Read the model definition and answer for the solid it produces. Units are mm, in the model's axes. Coordinates: 2 decimals unless noted, no trailing zeros. Loops run counter-clockwise (first coordinate to the right, second up) from the corner with the lowest first, then second, coordinate; pieces in that order, holes last. Notation, with made-up numbers: M 70,5 L 127,5 A9 cw 127,17 Z; hole C -29,-19.75 d10. An arc over 180 degrees is marked long. Use one line per item in the form item = value. Start each with the question number.
1. A flat-ended cylindrical pin translates along its axis: pin 1 (4 mm diameter, centred on x = 0, y = 0, fed in from +Z) (3 decimals). Find the tip coordinate at first contact, or state that the pin passes through.
2. The part is cut by section B-B (y = 0). Give the vertices of the cut face in (x, z) (1 decimal), plus the area to 3 significant figures.
3. The part is cut by section A-A (x = 0). Give the vertices of the cut face in (y, z) (1 decimal), plus the area to 3 significant figures.
4. Find the intervals of material crossed by probe 1 along Y at (x, z) = (0, 0.35) (3 decimals); probe 2 along Y at (x, z) = (179, 1.1); probe 3 along X at (y, z) = (-1.5, 0.5), in increasing order. Write a range as [from, to].
5. The part is cut by section D-D (x = 123). Give the vertices of the cut face in (y, z).
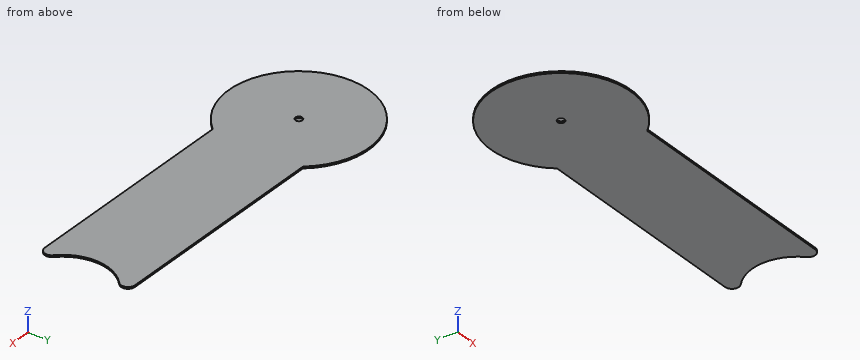
from build123d import *

# Parameters (mm, degrees)
SKETCH1_R           = 3.175
BOSS_EXTRUDE1_DEPTH = 1.5875


with BuildPart() as part:
    # Sketch1 → Boss-Extrude1 (new body)
    with BuildSketch(Plane.XY):
        with BuildLine():
            Line((247.146000248, -40.9575), (48.525593183, -40.9575))
            ThreePointArc((48.525593183, -40.9575), (-63.5, 0), (48.525593183, 40.9575))
            Line((48.525593183, 40.9575), (247.146000248, 40.9575))
            ThreePointArc((247.146000248, 40.9575), (253.054475846, 36.933959995), (251.475396188, 29.962197987))
            ThreePointArc((251.475396188, 29.962197987), (238.4425, 0), (251.475396188, -29.962197987))
            ThreePointArc((251.475396188, -29.962197987), (253.054475846, -36.933959995), (247.146000248, -40.9575))
        make_face()
        Circle(SKETCH1_R, mode=Mode.SUBTRACT)
    extrude(amount=BOSS_EXTRUDE1_DEPTH)


solid = part.part
Computed values:
q1.pin_1 = through
q2.outline = M -63.5,0 L -3.2,0 L -3.2,1.6 L -63.5,1.6 Z; M 3.2,0 L 238.4,0 L 238.4,1.6 L 3.2,1.6 Z
q2.area = 469 mm²
q3.outline = M -63.5,0 L -3.2,0 L -3.2,1.6 L -63.5,1.6 Z; M 3.2,0 L 63.5,0 L 63.5,1.6 L 3.2,1.6 Z
q3.area = 192 mm²
q4.probe_1 = [-63.5, -3.175], [3.175, 63.5]
q4.probe_2 = [-40.96, 40.96]
q4.probe_3 = [-63.48, -2.8], [2.8, 238.47]
q5.outline = M -40.96,0 L 40.96,0 L 40.96,1.59 L -40.96,1.59 Z
